```python
from build123d import *

# Parameters (mm, degrees)
SKETCH1_W           = 111
SKETCH1_H           = 28
SKETCH1_W_2         = 4.5
SKETCH1_H_2         = 2
BOSS_EXTRUDE1_DEPTH = 1
FILLET1_R           = 1


with BuildPart() as part:
    # Sketch1 → Boss-Extrude1 (new, symmetric)
    with BuildSketch(Plane.XY):
        Rectangle(SKETCH1_W, SKETCH1_H)
        with Locations((0, -15)):
            Rectangle(SKETCH1_W_2, SKETCH1_H_2)
        with Locations((27.2, 15)):
            Rectangle(SKETCH1_W_2, SKETCH1_H_2)
        with Locations((-27.2, 15)):
            Rectangle(SKETCH1_W_2, SKETCH1_H_2)
        with Locations((-48.9, -15)):
            Rectangle(SKETCH1_W_2, SKETCH1_H_2)
        with Locations((48.9, -15)):
            Rectangle(SKETCH1_W_2, SKETCH1_H_2)
    extrude(amount=BOSS_EXTRUDE1_DEPTH, both=True)

    # Fillet1
    fillet1_edges = [part.edges().sort_by_distance(p)[0] for p in [
        (55.5, -14, 0),
        (2.25, -16, 0),
        (-2.25, -16, 0),
        (-55.5, -14, 0),
        (-55.5, 14, 0),
        (-29.45, 16, 0),
        (-24.95, 16, 0),
        (24.95, 16, 0),
        (29.45, 16, 0),
        (55.5, 14, 0),
        (-51.15, -16, 0),
        (-46.65, -16, 0),
        (46.65, -16, 0),
        (51.15, -16, 0),
    ]]
    fillet(fillet1_edges, radius=FILLET1_R)


solid = part.part
```
Design review of the part built by this model. Coordinates are the model's own, in mm. A direction names the side the tool comes from. Round coordinates to 2 decimals unless told otherwise and drop trailing zeros. Order: outer loops, then holes, each group sorted by start corner. A loop starts at its lowest first (then second) coordinate and runs counter-clockwise, first axis right, second up. Notation, with made-up numbers: (-34, 16.25) - (-10, 16.25) arc R23 cw to (-10, 29.25) - close; hole circle Ø6 at (51.25, 39.5). An arc over 180 degrees is marked (long way). Return JSON: item names as keys, results as strings.
Q1. For pin 1 Ø0.6 at (x, z) = (2.5, -0.5) entering from +Y; pin 2 Ø0.5 at (y, z) = (-14.5, 0) entering from +X; pin 3 Ø0.5 at (y, z) = (14.5, -0.5) entering from -X, all flat-tipped, find the tip position at first contact; note any pin that passes through.
Computed values:
{"pin 1": "stops at y = 14", "pin 2": "stops at x = 51.15", "pin 3": "stops at x = -29.45"}
Q2. Wall thickness on L1, parallel to Y at x = 41.5, z = 0.5; L2, parallel to Y at x = 49, z = -0.6: over which ranges is each line inside the solid? List them lowest first. Write a range as [from, to].
Computed values:
{"L1": "y = [-14, 14]", "L2": "y = [-16, 14]"}
Q3. Machinability: for faces 1 (the flat face through (-42, 14, 0)), 2 (the flat face through (53, -14, 0)), 3 (the flat face through (-53, -14, 0)), 4 (the flat face through (42, 14, 0)), 5 (the flat face through (24, -14, 0)), which of the approach directions +Z, -Z, +X, -X, +Y, -Y give a long, thin tool a straight path to every point of the face, cutting with its end or side? Answer none if there is none.
Computed values:
{"face 1": "+Z, -Z, -X, +Y", "face 2": "+Z, -Z, +X, -Y", "face 3": "+Z, -Z, -X, -Y", "face 4": "+Z, -Z, +X, +Y", "face 5": "+Z, -Z, -Y"}
Q4. Consider section A-A on x = -37.5. Write out the cut boundary in (y, z), plus the area to 3 significant figures.
Computed values:
{"outline": "(-14, -1) - (14, -1) - (14, 1) - (-14, 1) - close", "area": "56.0 mm2"}
Q5. The part is to be moulded in two halves that separate along X. For faces 6 (the flat face through (55.5, 0, 0)), 7 (the flat face through (-25, -14, 0)), 8 (the flat face through (0, 14, 0)), 9 (the flat face through (27, 16, 0)), say which applies: pulls with the +X half, pulls with the -X half, needs draft (parallel to the pull), parting line crosses it, or undercut.
Computed values:
{"face 6": "pulls with the +X half", "face 7": "undercut", "face 8": "undercut", "face 9": "needs draft"}
